Work out the finished part from the listing and answer in its coordinate system (mm). A direction names the side the tool comes from. Coordinates: 2 decimals unless noted, no trailing zeros. Loops run counter-clockwise (first coordinate to the right, second up) from the corner with the lowest first, then second, coordinate; pieces in that order, holes last. Notation, with made-up numbers: (-19.5, -20.75) -> (30.5, -20.75) arc R11 ccw to (30.5, -12.75) -> close; hole circle Ø8 at (14.5, 34). An arc over 180 degrees is marked (long way). Answer as CSV lines item,"result".
Autodesk Inventor part; units mm, degrees
ref_plane "YZ Plane" through (0, 0, 0) normal (1, 0, 0) x (0, 1, 0)
ref_plane "XZ Plane" through (0, 0, 0) normal (0, 1, 0) x (-1, 0, 0)
ref_plane "XY Plane" through (0, 0, 0) normal (0, 0, 1) x (1, 0, 0)
sketch "Sketch1" plane through (0, 0, 0) normal (0, 0, 1) x (1, 0, 0)
  line L0 (0, 0) -> (50.8, 0)
  line L1 (50.8, 0) -> (50.8, -3.175)
  line L2 (3.175, -50.8) -> (0, -50.8)
  line L3 (0, -50.8) -> (0, 0)
  line L4 (3.175, -50.8) -> (3.175, -3.175)
  line L5 (3.175, -3.175) -> (50.8, -3.175)
  dimension "d0" = 50.8
  dimension "d1" = 50.8
  dimension "d2" = 3.175
  dimension "d3" = 3.175
extrude "Extrusion1" add sketch "Sketch1" along normal blind 50.8
sketch "Sketch2" plane through (0, -50.8, 0) normal (-1, 0, 0) x (0, 0, 1)
  circle A0 centre (22.5814, 25.4) radius 14.2875
  line L0 (0, 50.8) -> (50.8, 50.8)
  line L1 (0, 0) -> (50.8, 0)
  dimension "d6" = 25.4
  dimension "d7" = 25.4
  dimension "d8" = 28.575
extrude "Extrusion2" cut sketch "Sketch2" against normal through all
properties part number "Lbracket" material "Aluminum 6061"
(1) A cutting plane is placed at C-C, the plane z = 5. Write down the section's boundary in (x, y) (3 decimals), and give its area (4 significant figures).
Computed values:
outline,"(0, -50.8) -> (3.175, -50.8) -> (3.175, -3.175) -> (50.8, -3.175) -> (50.8, 0) -> (0, 0) -> close"
area,"312.5 mm2"
(2) A cutting plane is placed at D-D, the plane y = -17. Write down the section's boundary in (x, z) (3 decimals), and give its area (3 significant figures).
Computed values:
outline,"(0, 0) -> (3.175, 0) -> (3.175, 11.024) -> (0, 11.024) -> close; (0, 34.139) -> (3.175, 34.139) -> (3.175, 50.8) -> (0, 50.8) -> close"
area,"87.9 mm2"
(3) For a pull along Y with two mould halves and no side action, classify faces 3 (the face through (50.8, -2, 25)), 4 (the face through (25, 0, 25)), 5 (the face through (1.57, -13.35, 30.26)) as pulls with the +Y half, pulls with the -Y half, needs draft (parallel to the pull), parting line crosses it, or undercut.
Computed values:
face 3,"needs draft"
face 4,"pulls with the +Y half"
face 5,"undercut"
(4) A cutting plane is placed at A-A, the plane y = -25.4. Write down the section's boundary in (x, z) (3 decimals).
Computed values:
outline,"(0, 0) -> (3.175, 0) -> (3.175, 8.294) -> (0, 8.294) -> close; (0, 36.869) -> (3.175, 36.869) -> (3.175, 50.8) -> (0, 50.8) -> close"
(5) Consider line 1 along Z through (x, y) = (2, -25); line 2 along Y through (x, z) = (31, 9) (3 decimals); line 3 along X through (y, z) = (-20, 2) (3 decimals). Determine where each line is inside the solid, lowest interval first.
Computed values:
line 1,"0 to 8.3, 36.86 to 50.8"
line 2,"-3.175 to 0"
line 3,"0 to 3.175"
(6) A cutting plane is placed at B-B, the plane z = 30. Write down the section's boundary in (x, y) (3 decimals), and give its area (3 significant figures).
Computed values:
outline,"(0, -50.8) -> (3.175, -50.8) -> (3.175, -37.611) -> (0, -37.611) -> close; (0, -13.189) -> (3.175, -13.189) -> (3.175, -3.175) -> (50.8, -3.175) -> (50.8, 0) -> (0, 0) -> close"
area,"235 mm2"
(7) Which of the six approach directions +Z, -Z, +X, -X, +Y, -Y give full straight-line access (tool end or side, diameter ignored) to faces 1 (the face through (3.175, -38, 31)), 2 (the face through (3, -14, 0))?
Computed values:
face 1,"+Z, -Z, +X, -Y"
face 2,"-Z, +X, -X, +Y, -Y"
(8) Flat-ended cylindrical pins translate along their axes: pin 1 Ø4 at (x, y) = (6, -36) entering from +Z; pin 2 Ø24 at (y, z) = (-28, 20) entering from +X (3 decimals); pin 3 Ø5 at (x, z) = (12.5, 6) entering from -Y (3 decimals). Find the tip coordinate at first contact, or state that the pin passes through.
Computed values:
pin 1,"through"
pin 2,"x = 3.175"
pin 3,"y = -3.175"
